```python
from build123d import *

# Parameters (mm, degrees)
DODANIE_WYCI_GNI_CIE1_DEPTH = 45
DODANIE_WYCI_GNI_CIE3_DEPTH = 22.5


with BuildPart() as part:
    # Szkic1 → Dodanie-wyciągnięcie1 (new, symmetric)
    with BuildSketch(Plane.XY):
        with BuildLine():
            Line((67.5, 0), (-67.5, 0))
            Line((-67.5, 0), (-67.5, 45))
            Line((-67.5, 45), (-45, 45))
            Line((-45, 45), (-45, 100))
            ThreePointArc((-45, 100), (0, 145), (45, 100))
            Line((45, 100), (45, 45))
            Line((45, 45), (67.5, 45))
            Line((67.5, 45), (67.5, 0))
        make_face()
        with BuildLine():
            Line((35, 35), (35, 100))
            ThreePointArc((35, 100), (0, 135), (-35, 100))
            Line((-35, 100), (-35, 35))
            Line((-35, 35), (-57.5, 35))
            Line((-57.5, 35), (-57.5, 10))
            Line((-57.5, 10), (57.5, 10))
            Line((57.5, 10), (57.5, 35))
            Line((57.5, 35), (35, 35))
        make_face(mode=Mode.SUBTRACT)
    extrude(amount=DODANIE_WYCI_GNI_CIE1_DEPTH, both=True)

    # Szkic2 → Dodanie-wyciągnięcie3 (add)
    with BuildSketch(Plane(origin=(67.5, 0, 0), x_dir=(0, 0, -1), z_dir=(1, 0, 0))):
        with BuildLine():
            Line((-18, 45), (18, 45))
            Line((18, 45), (18, 65))
            ThreePointArc((18, 65), (0, 83), (-18, 65))
            Line((-18, 65), (-18, 45))
        make_face()
    extrude(amount=-DODANIE_WYCI_GNI_CIE3_DEPTH)


solid = part.part
```
Check sheet for the modelled part. Datum: model origin and axes. Units: mm. A direction names the side the tool comes from. Give positions to 0.01 mm unless a question says otherwise; leave off trailing zeros. Order: outer loops, then holes, each group sorted by start corner. A loop starts at its lowest first (then second) coordinate and runs counter-clockwise, first axis right, second up. Notation, with made-up numbers: (1, -33) -> (23, -33) arc R21 cw to (23, -27) -> close; hole circle Ø9 at (65.5, 73). An arc over 180 degrees is marked (long way). Use CSV: the item, a comma, the result in double quotes. Start each with the question number.
1) Set-up check for faces 5 (the face through (56, 83, 0)), 6 (the face through (56, 55, -18)), 7 (the face through (-45, 72, 1)): record each of +Z, -Z, +X, -X, +Y, -Y from which the full face is reachable in a straight line by a thin tool's end or side.
2) Mould release check, pull along Y, two halves, no side actions. Record for faces 1 (the face through (56, 45, 32)), 2 (the face through (57.5, 22, 1)), 3 (the face through (-46, 35, 1)), 4 (the face through (56, 55, 18)): released by +Y, released by -Y, zero draft, split by the parting line, or undercut.
3) Material ranges on line 1 (X direction, y = 26, z = -19); line 2 (X direction, y = 81.5, z = -15); line 3 (Y direction, x = 5, z = -9.5), recorded low to high. Write a range as from..to.
4) Go/stop test with flat-tipped pins: P1, Ø18, axis at x = -61.5, z = -17.5, coming from the +Y side; P2, Ø10, axis at x = 59, y = 53, coming from the -Z side. Record where each tip stops, or that it passes through.
5) Sectioned sample at C-C, the plane x = 0. Record the boundary of the cut face in (y, z), plus the area to 3 significant figures.
6) Sectioned sample at A-A, the plane y = 88. Record the boundary of the cut face in (x, z), plus the area to 3 significant figures.
7) Sectioned sample at B-B, the plane z = 0. Record the boundary of the cut face in (x, y).
8) Sectioned sample at D-D, the plane y = 57.5. Record the boundary of the cut face in (x, z).
Recorded:
1,face 5,"+X, +Y"
1,face 6,"-Z, +X, +Y"
1,face 7,"+Z, -Z, -X, +Y"
2,face 1,"released by +Y"
2,face 2,"undercut"
2,face 3,"undercut"
2,face 4,"zero draft"
3,line 1,"-67.5..-57.5, 57.5..67.5"
3,line 2,"-45..-35, 35..45"
3,line 3,"0..10, 134.64..144.72"
4,P1,"y = 45"
4,P2,"z = -18"
5,outline,"(0, -45) -> (10, -45) -> (10, 45) -> (0, 45) -> close; (135, -45) -> (145, -45) -> (145, 45) -> (135, 45) -> close"
5,area,"1,800 mm2"
6,outline,"(-45, -45) -> (-35, -45) -> (-35, 45) -> (-45, 45) -> close; (35, -45) -> (45, -45) -> (45, 45) -> (35, 45) -> close"
6,area,"1,800 mm2"
7,outline,"(-67.5, 0) -> (67.5, 0) -> (67.5, 83) -> (45, 83) -> (45, 100) arc R45 ccw to (-45, 100) -> (-45, 45) -> (-67.5, 45) -> close; hole (-57.5, 10) -> (57.5, 10) -> (57.5, 35) -> (35, 35) -> (35, 100) arc R35 ccw to (-35, 100) -> (-35, 35) -> (-57.5, 35) -> close"
8,outline,"(-45, -45) -> (-35, -45) -> (-35, 45) -> (-45, 45) -> close; (35, -45) -> (45, -45) -> (45, -18) -> (67.5, -18) -> (67.5, 18) -> (45, 18) -> (45, 45) -> (35, 45) -> close"
